Work out the finished part from the listing and answer in its coordinate system (mm). A direction names the side the tool comes from. Coordinates: 2 decimals unless noted, no trailing zeros. Loops run counter-clockwise (first coordinate to the right, second up) from the corner with the lowest first, then second, coordinate; pieces in that order, holes last. Notation, with made-up numbers: (68, 75) -> (84, 75) arc R18 ccw to (84, 107) -> close; hole circle Ø4 at (82, -32.5). An arc over 180 degrees is marked (long way). One line per question, with ' | ' between items.
```python
from build123d import *

# Parameters (mm, degrees)
F0_R      = 13
F1_DEPTH  = 25
F3_R      = 2.5
F7_ANGLE  = 90
F2_R      = 13
F2_R_2    = 11.8
F10_DEPTH = 10


with BuildPart() as f1:
    # F0 (on Top) → F1 (new body)
    with BuildSketch(Plane.XY):
        Circle(F0_R)
    extrude(amount=F1_DEPTH)

    # F8 (on Front) → F9 (revolve)
    with BuildSketch(Plane.XZ):
        with BuildLine():
            Line((0, 0), (0, -13))
            ThreePointArc((0, -13), (9.1923881554, -9.1923881554), (13, 0))
            Line((13, 0), (0, 0))
        make_face()
    revolve(axis=Axis((0, 0, 0), (0, 0, 1)))

    # F2 (on face) → F10 (cut)
    with BuildSketch(Plane.XY.offset(25)):
        Circle(F2_R)
        Circle(F2_R_2, mode=Mode.SUBTRACT)
    extrude(amount=-F10_DEPTH, mode=Mode.SUBTRACT)


with BuildPart() as f5:
    # F3 (on Front) → F5 (revolve)
    with BuildSketch(Plane.XZ):
        with Locations((-50, 50)):
            Circle(F3_R)
    revolve(axis=Axis((-130, 0, 0), (0, 0, 1)))


with BuildPart() as f5_1:
    # F6: moved
    add(f5.part.moved(Location((50, 0, 0))))


with BuildPart() as f5_2:
    # F7: moved
    add(f5_1.part.rotate(Axis((-88.6065643281, 0, 50), (-1, 0, 0)), F7_ANGLE))


with BuildPart() as f1_1:
    add(f1.part)

    # F11: cut F5
    add(f5_2.part, mode=Mode.SUBTRACT)


solid = f1_1.part
```
1) Find section B-B (x = 0). Write down the section's boundary in (y, z).
Check values:
outline: (-13, 0) arc R13 ccw to (13, 0) -> (13, 15) -> (11.8, 15) -> (11.8, 25) -> (-11.8, 25) -> (-11.8, 15) -> (-13, 15) -> close
2) Find section A-A (y = 0). Write down the section's boundary in (x, z), plus the area to 3 significant figures.
Check values:
outline: (-13, 0) arc R13 ccw to (13, 0) -> (13, 15) -> (11.8, 15) -> (11.8, 25) -> (-1.38, 25) arc R82.5 cw to (-13, 1.86) -> close; (-13, 11.05) arc R77.5 ccw to (-6.64, 25) -> (-11.8, 25) -> (-11.8, 15) -> (-13, 15) -> close | area: 788 mm^2
3) For faces 1 (the face through (-11.79, 0.52, 20.07)), 2 (the face through (0, 0, 25)), determine the directions among +Z, -Z, +X, -X, +Y, -Y from which every point of the face is accessible in a straight line to the end or side of a thin tool.
Check values:
face 1: +Z | face 2: +Z, +X, -X, +Y, -Y
4) Find the intervals of material crossed by line 1 along Y through (x, z) = (-6.5, 22.5); line 2 along Y through (x, z) = (-0.5, 13.5); line 3 along Z through (x, y) = (6.5, 2.25), in increasing order.
Check values:
line 1: y = -9.85 to -1.98, 1.98 to 9.85 | line 2: y = -12.99 to 12.99 | line 3: z = -11.03 to 25
5) Flat-ended cylindrical pins translate along their axes: pin 1 (4 mm diameter, centred on y = -7.5, z = -3, fed in from +X); pin 2 (3 mm diameter, centred on y = -0.5, z = -5, fed in from -X); pin 3 (8 mm diameter, centred on y = 10, z = -3, fed in from +X). Find the tip coordinate at first contact, or state that the pin passes through.
Check values:
pin 1: stops at x = 11.49 | pin 2: stops at x = -12.51 | pin 3: stops at x = 11.29
6) Find section C-C (y = 11.25). Write down the section's boundary in (x, z), plus the area to 3 significant figures.
Check values:
outline: (-6.51, 0) arc R6.51 ccw to (6.51, 0) -> (6.51, 15) -> (3.56, 15) -> (3.56, 25) -> (-3.56, 25) -> (-3.56, 15) -> (-6.51, 15) -> close | area: 333 mm^2
7) Find section D-D (z = -4.5). Write down the section's boundary in (x, y), plus the area to 3 significant figures.
Check values:
outline: circle Ø24.39 at (0, 0) | area: 467 mm^2
